Autodesk Fusion 360 part; units mm, degrees
sketch "Sketch1" plane through (0, 0, 0) normal (0, 1, 0) x (1, 0, 0)
  circle A0 centre (0, 0) radius 25
  dimension "d1" = 50
extrude "Extrude1" add sketch "Sketch1" along normal blind 10
sketch "Sketch2" plane through (0, 10, 0) normal (0, 1, 0) x (-1, 0, 0)
  circle A0 centre (0, 0) radius 25
  circle A1 centre (0, 0) radius 21
  dimension "d4" = 42
extrude "Extrude2" cut sketch "Sketch2" against normal blind 5 contours A1
sketch "Sketch3" plane through (0, 5, 0) normal (0, 1, 0) x (-1, 0, 0)
  circle A0 centre (0, 0) radius 21
  circle A1 centre (0, 0) radius 5
  dimension "d7" = 10
extrude "Extrude3" cut sketch "Sketch3" against normal through all contours A1
ref_plane "WorkPlane1" through (-8.5505, 3.5882, -23.4923) normal (-0.342, 0, -0.9397) x (0.9397, 0, -0.342)
sketch "Sketch4" plane through (-8.5505, 3.5882, -23.4923) normal (-0.342, 0, -0.9397) x (0.9397, 0, -0.342)
  line L0 (-19.8743, 2.2343) -> (20.1257, 2.2343)
  line L1 (20.1257, 2.2343) -> (20.1257, -5.7657)
  line L2 (20.1257, -5.7657) -> (-19.8743, -5.7657)
  line L3 (-19.8743, -5.7657) -> (-19.8743, 2.2343)
  line L4 (-19.8743, 2.2343) -> (20.1257, -5.7657) construction
  line L5 (20.1257, 2.2343) -> (-19.8743, -5.7657) construction
  point P0 (0.1257, -1.7657)
  dimension "d10" = 40
  dimension "d11" = 8
extrude "Extrude4" add sketch "Sketch4" along normal blind 50 and the other way blind 17
extrude "Extrude5" cut 1 faces at (-8.2808, 9.3539, -12.2547) along direction (0, -1, 0) blind 4
extrude "Extrude6" add 1 faces at (-8.2808, 5.3539, -12.2547) along direction (0, -1, 0) blind 5
extrude "Extrude7" cut 1 faces at (-8.2808, 5.3539, -12.2547) along direction (0, -1, 0) blind 0.354
extrude "Extrude8" add 1 faces at (-19.2688, 6.6872, -72.8001) along direction (-0.34202, 0, -0.939693) blind 10
sketch "Sketch5" plane through (0, 9.3539, 0) normal (0, 1, 0) x (-1, 0, 0)
  arc A0 (-13.8395, -20.8199) -> (23.8629, -7.4541) centre (0, 0) ccw
  line L0 (-13.8395, -20.8199) -> (10.1597, -86.757)
  line L1 (10.1597, -86.757) -> (47.7474, -73.0762)
  line L2 (47.7474, -73.0762) -> (23.8629, -7.4541)
  line L3 (10.1597, -86.757) -> (6.7395, -77.36)
  line L4 (34.9302, -67.0994) -> (28.0898, -48.3056)
  line L5 (28.0898, -48.3056) -> (-0.1009, -58.5662)
  line L6 (34.9302, -67.0994) -> (6.7395, -77.36)
  dimension "d24" = 10
  dimension "d26" = 20
extrude "Extrude9" cut sketch "Sketch5" against normal through all contours L0 L4 L5 L6
extrude "Extrude10" add 1 faces at (-11.5472, 9.3539, -43.6568) along direction (0, 1, 0) blind 5
extrude "Extrude11" add 1 faces at (-22.8793, 10, -5.8181) along direction (0, 1, 0) blind 5
extrude "Extrude12" add 1 faces at (-2.433, 5, -6.5632) along direction (0, 1, 0) blind 5
extrude "Extrude13" add 1 faces at (-8.2808, 4.9999, -12.2547) along direction (0, 1, 0) blind 5
extrude "Extrude14" cut 1 faces at (-18.6929, 10.0206, -51.7258) along direction (0.34202, 0, 0.939693) blind 20
hole "Hole1" at (-25.5993, 7.935, -81.1374) direction (0.342, 0, 0.9397) diameter 10 depth 14 tip angle 118
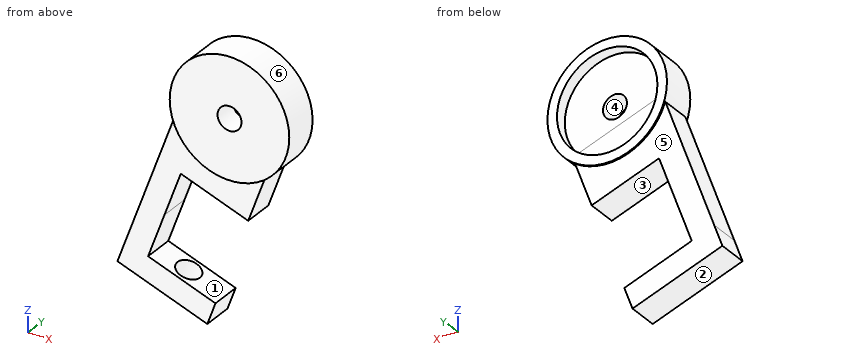
Can you work these out from the model? Positions are in its coordinate system, mm. Face numbers are marked on the shaded views. A direction names the side the tool comes from. Coordinates: 2 decimals unless noted, no trailing zeros. Write each loop counter-clockwise with the first axis right and the second up, starting at its lowest first coordinate (ties: lowest second). Pieces come first, ordered by that corner, then holes. Notation, with made-up numbers: (32.25, 20) -> (39.25, 20) arc R32 ccw to (39.25, 52) -> close; hole circle Ø8 at (35, 27.5). An arc over 180 degrees is marked (long way). Answer as CSV lines item,"result".
1) If I drill on line 1 (X direction, y = 11.4, z = 0); line 2 (Y direction, x = 0, z = -5.5); line 3 (Z direction, x = 5, y = 11.25), over which ranges is the centre line in solid material (lowest first)? Write a range as from..to.
Check result:
line 1,"-25..-21, 21..25"
line 2,"0..10"
line 3,"-39.07..-20.4, 20.4..24.49"
2) If we mould it in two halves opening along X, with no side actions, what happens to the marked faces 4, 5 and 6? For each: +X half, -X half, draft (parallel to the pull), parting line (faces both ways), or undercut.
Check result:
face 4,"undercut"
face 5,"draft"
face 6,"parting line"
3) If we section it at A-A on z = -33: Please give me the cut outline in (x, y).
Check result:
outline,"(-33.16, 1.35) -> (-22.52, 1.35) -> (-22.52, 14.35) -> (-33.16, 14.35) -> close; (-11.67, 1.35) -> (9.41, 1.35) -> (9.41, 14.35) -> (-11.67, 14.35) -> close"
4) If we section it at B-B on x = -8: Please give me the cut outline in (y, z).
Check result:
outline,"(0, -23.69) -> (1.35, -23.69) -> (1.35, -34.33) -> (14.35, -34.33) -> (14.35, -23.69) -> (15, -23.69) -> (15, -19.42) -> (10, -19.42) -> (10, 19.42) -> (15, 19.42) -> (15, 23.69) -> (0, 23.69) -> close; (1.35, -80.82) -> (14.35, -80.82) -> (14.35, -76.9) -> (1.35, -76.9) -> close"
5) On a 3-axis mill with a long thin cutter (end or side, diameter ignored), from which of +Z, -Z, +X, -X, +Y, -Y can I reach the whole of each face in a straight line? I mean the marked faces 1, 2 and 3. Say none if no direction works.
Check result:
face 1,"+X, +Y, -Y"
face 2,"-Z, -X, +Y, -Y"
face 3,"+Y, -Y"
6) If we section it at D-D on z = -2: Please give me the cut outline in (x, y).
Check result:
outline,"(-24.92, 0) -> (-4.58, 0) -> (-4.58, 10) -> (-20.9, 10) -> (-20.9, 15) -> (-24.92, 15) -> close; (4.58, 0) -> (24.92, 0) -> (24.92, 15) -> (20.9, 15) -> (20.9, 10) -> (4.58, 10) -> close"
7) Will these pins go through, and if not, where does the flat tip stop? P1, Ø4, axis at x = -18, z = -27, coming from the -Y side; P2, Ø8, axis at x = 14.5, z = -4, coming from the +Y side; P3, Ø1, axis at y = 6, z = -59.5, coming from the +X side; P4, Ø16, axis at x = -3.5, z = -14, coming from the +Y side.
Check result:
P1,"y = 1.35"
P2,"y = 10"
P3,"x = -31.98"
P4,"y = 15"
